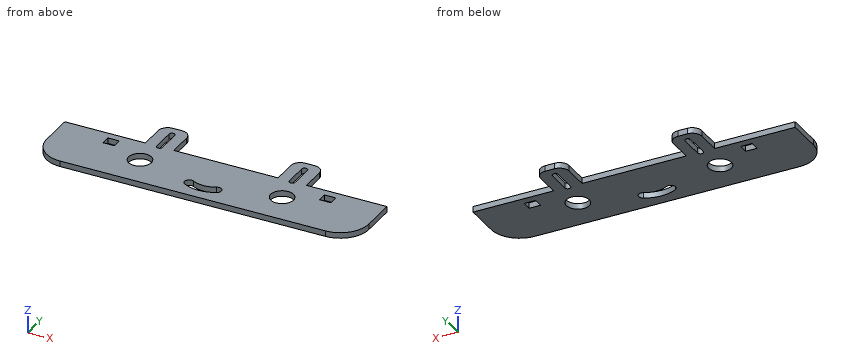
from build123d import *

# Parameters (mm, degrees)
BOSS_EXTRUDE1_DEPTH = 3
FILLET2_R           = 5
SKETCH3_R           = 6
CUT_EXTRUDE1_DEPTH  = 10
SKETCH4_W           = 6
SKETCH4_H           = 5
CUT_EXTRUDE2_DEPTH  = 10


with BuildPart() as part:
    # Sketch1 → Boss-Extrude1 (new body)
    with BuildSketch(Plane.XY):
        with BuildLine():
            Line((-103.55358225, -48), (-61.05358225, -48))
            Line((-61.05358225, -48), (-61.05358225, -30))
            Line((-61.05358225, -30), (-46.05358225, -30))
            Line((-46.05358225, -30), (-46.05358225, -48))
            Line((-46.05358225, -48), (8.94641775, -48))
            Line((8.94641775, -48), (8.94641775, -30))
            Line((8.94641775, -30), (23.94641775, -30))
            Line((23.94641775, -30), (23.94641775, -48))
            Line((23.94641775, -48), (66.44641775, -48))
            Line((66.44641775, -48), (66.44641775, -66.348486101))
            ThreePointArc((66.44641775, -66.348486101), (62.053019468, -76.955087819), (51.44641775, -81.348486101))
            Line((51.44641775, -81.348486101), (-88.55358225, -81.348486101))
            ThreePointArc((-88.55358225, -81.348486101), (-99.160183967, -76.955087819), (-103.55358225, -66.348486101))
            Line((-103.55358225, -66.348486101), (-103.55358225, -48))
        make_face()
        with BuildLine():
            Line((-55.05358225, -48.000000021), (-55.05358225, -35.500000021))
            ThreePointArc((-55.05358225, -35.500000021), (-53.55358225, -34.000000021), (-52.05358225, -35.500000021))
            Line((-52.05358225, -35.500000021), (-52.05358225, -48.000000021))
            ThreePointArc((-52.05358225, -48.000000021), (-53.55358225, -49.500000021), (-55.05358225, -48.000000021))
        make_face(mode=Mode.SUBTRACT)
        with BuildLine():
            Line((14.97417929, -48.006597652), (14.918685775, -35.506720833))
            ThreePointArc((14.918685775, -35.506720833), (16.412011771, -34.000076394), (17.918656211, -35.49340239))
            Line((17.918656211, -35.49340239), (17.974149726, -47.993279208))
            ThreePointArc((17.974149726, -47.993279208), (16.48082373, -49.499923648), (14.97417929, -48.006597652))
        make_face(mode=Mode.SUBTRACT)
    extrude(amount=BOSS_EXTRUDE1_DEPTH)

    # Fillet2
    fillet2_edges = [part.edges().sort_by_distance(p)[0] for p in [
        (-61.05358225, -30, 1.5),
        (-46.05358225, -30, 1.5),
        (8.94641775, -30, 1.5),
        (23.94641775, -30, 1.5),
    ]]
    fillet(fillet2_edges, radius=FILLET2_R)

    # Sketch3 → Cut-Extrude1 (cut)
    with BuildSketch(Plane.XY.offset(3)):
        with Locations((-56.05358225, -63)):
            Circle(SKETCH3_R)
        with Locations((18.94641775, -63)):
            Circle(SKETCH3_R)
        with BuildLine():
            ThreePointArc((-27.106412897, -73.26758291), (-18.643210609, -75.499770477), (-10.157587782, -73.354389499))
            ThreePointArc((-10.157587782, -73.354389499), (-9.163531348, -69.961477504), (-12.556443344, -68.967421071))
            ThreePointArc((-12.556443344, -68.967421071), (-18.617602506, -70.499836055), (-24.662746998, -68.905416364))
            ThreePointArc((-24.662746998, -68.905416364), (-28.06566322, -69.864666688), (-27.106412897, -73.26758291))
        make_face()
    extrude(amount=-CUT_EXTRUDE1_DEPTH, mode=Mode.SUBTRACT)

    # Sketch4 → Cut-Extrude2 (cut)
    with BuildSketch(Plane.XY.offset(3)):
        with Locations((38.567805477, -54.5)):
            Rectangle(SKETCH4_W, SKETCH4_H)
        with Locations((-75.674969976, -54.5)):
            Rectangle(SKETCH4_W, SKETCH4_H)
    extrude(amount=-CUT_EXTRUDE2_DEPTH, mode=Mode.SUBTRACT)


solid = part.part
Input: part model. Units: mm. Frame: model coordinates. Coordinates: 2 decimals unless noted, no trailing zeros. Loops run counter-clockwise (first coordinate to the right, second up) from the corner with the lowest first, then second, coordinate; pieces in that order, holes last.
(1) Section C-C on z = 2.35. Count the separate pieces of the cut face and the enclosed holes in it, then the cut area to 3 significant figures.
(2) Section A-A on y = -63. Return the cut outline in (x, z), then the cut area to 3 significant figures.
(3) Section B-B on x = -2. Return the cut outline in (y, z), then the cut area to 3 significant figures.
(4) Material intervals for probe 1 along X at (y, z) = (-53, 1.5); probe 2 along X at (y, z) = (-36.5, 0.65); probe 3 along Y at (x, z) = (-78, 2.7), sorted ascending.
(5) First-contact query: pin 1 Ø0.9 at (y, z) = (-38.5, 1) entering from -X; pin 2 Ø0.9 at (y, z) = (-44.5, 2) entering from +X; pin 3 Ø1.5 at (x, z) = (-76, 2) entering from +Y. Flat tips, straight axial feed; report the tip coordinate or a pass-through.
Data:
1. separate pieces: 1
1. enclosed holes: 7
1. area: 5,620 mm2
2. outline: (-103.55, 0) - (-62.05, 0) - (-62.05, 3) - (-103.55, 3) - close; (-50.05, 0) - (12.95, 0) - (12.95, 3) - (-50.05, 3) - close; (24.95, 0) - (66.45, 0) - (66.45, 3) - (24.95, 3) - close
2. area: 438 mm2
3. outline: (-81.35, 0) - (-48, 0) - (-48, 3) - (-81.35, 3) - close
3. area: 100 mm2
4. probe 1: x = -103.55 to -78.67, -72.67 to 35.57, 41.57 to 66.45
4. probe 2: x = -61.05 to -55.05, -52.05 to -46.05, 8.95 to 14.92, 17.92 to 23.95
4. probe 3: y = -81.35 to -57, -52 to -48
5. pin 1: stops at x = -61.05
5. pin 2: stops at x = 23.95
5. pin 3: stops at y = -48
